Check sheet for the modelled part. Datum: model origin and axes. Units: mm. Round coordinates to 2 decimals unless told otherwise and drop trailing zeros. Write each loop counter-clockwise with the first axis right and the second up, starting at its lowest first coordinate (ties: lowest second). Pieces come first, ordered by that corner, then holes.
Item 1: Cross-section at C-C on z = -140. Enter the section's corners in (x, y), plus the area to 3 significant figures.
Item 2: Cross-section at A-A on y = 1.35. Enter the section's corners in (x, z), plus the area to 3 significant figures.
Item 3: Material ranges on line 1 (Z direction, x = 203, y = 0.9); line 2 (X direction, y = 2.35, z = -142); line 3 (X direction, y = 4.25, z = -140.5), recorded low to high.
Item 4: Cross-section at B-B on x = 90.5. Enter the section's corners in (y, z), plus the area to 3 significant figures.
from build123d import *

# Parameters (mm, degrees)
BOSS_EXTRUDE1_DEPTH = 4.7625


with BuildPart() as part:
    # Sketch1 → Boss-Extrude1 (new body)
    with BuildSketch(Plane(origin=(0, 0, 0), x_dir=(1, 0, 0), z_dir=(0, 1, 0))):
        Polygon((152.4, 0), (0, 0), (0, 152.4), align=None)
        Polygon((120.65, 31.75), (152.4, 0), (350.901, 0), (350.901, 31.75), align=None)
    extrude(amount=BOSS_EXTRUDE1_DEPTH)


solid = part.part
Response values:
1. outline: (0, 0) - (12.4, 0) - (12.4, 4.76) - (0, 4.76) - close
1. area: 59.1 mm2
2. outline: (0, -152.4) - (120.65, -31.75) - (350.9, -31.75) - (350.9, 0) - (0, 0) - close
2. area: 18,400 mm2
3. line 1: z = -31.75 to 0
3. line 2: x = 0 to 10.4
3. line 3: x = 0 to 11.9
4. outline: (0, -61.9) - (4.76, -61.9) - (4.76, 0) - (0, 0) - close
4. area: 295 mm2
